from build123d import *

# Parameters (mm, degrees)
SKETCH1_W           = 11.699975178
SKETCH1_H           = 11.699996949
SKETCH1_W_2         = 11.699990436
SKETCH1_H_2         = 11.699981689
SKETCH1_W_3         = 11.699990437
SKETCH1_H_3         = 11.699975177
SKETCH1_W_4         = 11.699981689
SKETCH1_H_4         = 11.699990436
BOSS_EXTRUDE1_DEPTH = 1955.8


with BuildPart() as part:
    # Sketch1 → Boss-Extrude1 (new body)
    with BuildSketch(Plane.XY):
        Polygon((22.500515052, 22.499297556), (-22.499484399, 22.499298105), (-22.499484948, -22.500701346), (-4.249491942, -22.500701568), (-4.249491942, -22.200733242), (-4.24949208, -18.000719999), (-6.799479919, -18.000719999), (-6.799480207, -9.200732353), (-4.799480391, -7.200732362), (4.800525817, -7.200732047), (6.8005258, -9.200731855), (6.800526088, -18.000720263), (4.250507877, -18.000720263), (4.250508015, -22.200733153), (4.250508015, -22.500701672), (22.500514502, -22.500701895), (22.500514725, -4.250714302), (22.200520351, -4.250714302), (18.000507108, -4.25071444), (18.000507108, -6.800702279), (9.200519462, -6.800702567), (7.200519471, -4.800702751), (7.200519156, 4.799303458), (9.200518964, 6.79930344), (18.000507424, 6.799303729), (18.000507424, 4.249285514), (22.200520261, 4.249285652), (22.500514829, 4.249285652), align=None)
        with BuildLine():
            Line((-4.249491247, 17.999291576), (-4.249490956, 22.199304807))
            Line((-4.249490956, 22.199304807), (-3.949472548, 22.199304807))
            Line((-3.949472548, 22.199304807), (-3.481695222, 21.73152644))
            ThreePointArc((-3.481695222, 21.73152644), (-2.670636178, 21.189593132), (-1.713926324, 20.999291428))
            Line((-1.713926324, 20.999291428), (1.714975167, 20.999291428))
            ThreePointArc((1.714975167, 20.999291428), (2.671722509, 21.189608628), (3.482801459, 21.731583767))
            Line((3.482801459, 21.731583767), (3.950490798, 22.199304487))
            Line((3.950490798, 22.199304487), (4.250509108, 22.199304487))
            Line((4.250509108, 22.199304487), (4.250508817, 17.999291575))
            Line((4.250508817, 17.999291575), (6.800527063, 17.999291575))
            Line((6.800527063, 17.999291575), (6.800526453, 9.199302988))
            Line((6.800526453, 9.199302988), (4.800526064, 7.199302969))
            Line((4.800526064, 7.199302969), (-4.799479817, 7.199303635))
            Line((-4.799479817, 7.199303635), (-6.799479854, 9.199304042))
            Line((-6.799479854, 9.199304042), (-6.799479244, 17.999291576))
            Line((-6.799479244, 17.999291576), (-4.249491247, 17.999291576))
        make_face(mode=Mode.SUBTRACT)
        with BuildLine():
            Line((-22.199510888, 4.249285566), (-17.999497356, 4.249285704))
            Line((-17.999497356, 4.249285704), (-17.999497356, 6.79927354))
            Line((-17.999497356, 6.79927354), (-9.199509947, 6.799273828))
            Line((-9.199509947, 6.799273828), (-7.199509956, 4.799274012))
            Line((-7.199509956, 4.799274012), (-7.199509641, -4.800732197))
            Line((-7.199509641, -4.800732197), (-9.199509449, -6.800732179))
            Line((-9.199509449, -6.800732179), (-17.99949762, -6.800732468))
            Line((-17.99949762, -6.800732468), (-17.99949762, -4.250714253))
            Line((-17.99949762, -4.250714253), (-22.199510799, -4.250714391))
            Line((-22.199510799, -4.250714391), (-22.199510799, -3.950696126))
            Line((-22.199510799, -3.950696126), (-21.731790056, -3.48300681))
            ThreePointArc((-21.731790056, -3.48300681), (-21.189814855, -2.671927844), (-20.999497617, -1.71518046))
            Line((-20.999497617, -1.71518046), (-20.999497617, 1.713721031))
            ThreePointArc((-20.999497617, 1.713721031), (-21.189799286, 2.670430863), (-21.731732544, 3.481489907))
            Line((-21.731732544, 3.481489907), (-22.199510888, 3.949267256))
            Line((-22.199510888, 3.949267256), (-22.199510888, 4.249285566))
        make_face(mode=Mode.SUBTRACT)
        with Locations((-14.649542346, -14.650709384)):
            Rectangle(SKETCH1_W, SKETCH1_H, mode=Mode.SUBTRACT)
        with Locations((14.65050626, -14.650767962)):
            Rectangle(SKETCH1_W_2, SKETCH1_H_2, mode=Mode.SUBTRACT)
        with BuildLine():
            Line((-3.181457266, -4.596908447), (-4.595670829, -3.182694885))
            Line((-4.595670829, -3.182694885), (-3.26221457, -1.849238626))
            ThreePointArc((-3.26221457, -1.849238626), (-3.749476751, -0.00071437), (-3.26221457, 1.847809887))
            Line((-3.26221457, 1.847809887), (-4.595670829, 3.181266146))
            Line((-4.595670829, 3.181266146), (-3.181457266, 4.595479708))
            Line((-3.181457266, 4.595479708), (-1.848001007, 3.262023449))
            ThreePointArc((-1.848001007, 3.262023449), (0.000523249, 3.74928563), (1.849047505, 3.262023449))
            Line((1.849047505, 3.262023449), (3.182503764, 4.595479708))
            Line((3.182503764, 4.595479708), (4.596717327, 3.181266146))
            Line((4.596717327, 3.181266146), (3.263261068, 1.847809887))
            ThreePointArc((3.263261068, 1.847809887), (3.750523249, -0.00071437), (3.263261068, -1.849238626))
            Line((3.263261068, -1.849238626), (4.596717327, -3.182694885))
            Line((4.596717327, -3.182694885), (3.182503764, -4.596908447))
            Line((3.182503764, -4.596908447), (1.849047505, -3.263452188))
            ThreePointArc((1.849047505, -3.263452188), (0.000523249, -3.75071437), (-1.848001007, -3.263452188))
            Line((-1.848001007, -3.263452188), (-3.181457266, -4.596908447))
        make_face(mode=Mode.SUBTRACT)
        with Locations((-14.64949028, 14.649335967)):
            Rectangle(SKETCH1_W_3, SKETCH1_H_3, mode=Mode.SUBTRACT)
        with Locations((14.650561583, 14.6492839)):
            Rectangle(SKETCH1_W_4, SKETCH1_H_4, mode=Mode.SUBTRACT)
    extrude(amount=BOSS_EXTRUDE1_DEPTH)


solid = part.part
Check sheet for the modelled part. Datum: model origin and axes. Units: mm. Give positions to 0.01 mm unless a question says otherwise; leave off trailing zeros. Use a Markdown table: item, result. Add a question column.
Q1. Sectioned sample at A-A, the plane z = 1232.5. Give the number of separate pieces and of enclosed holes in the cut face, then the cut area to 3 significant figures.
Q2. Go/stop test with flat-tipped pins: pin 1 (4 mm diameter, centred on x = 5, y = 17.5, fed in from -Z); pin 2 (4 mm diameter, centred on y = 0.5, z = 1364, fed in from +X). Record where each tip stops, or that it passes through.
Q3. Scan lines: line 1 along Y through (x, z) = (-2.5, 138.5); line 2 along X through (y, z) = (19, 223); line 3 along X through (y, z) = (10.5, 1129.5). Record each from-to range of solid material in increasing order. Write a range as [from, to].
Verdict:
| question | item | result |
|---|---|---|
| 1 | separate pieces | 1 |
| 1 | enclosed holes | 7 |
| 1 | area | 715 mm^2 |
| 2 | pin 1 | z = 0 |
| 2 | pin 2 | x = 7.2 |
| 3 | line 1 | [-7.2, -3.92], [3.91, 7.2], [21.13, 22.5] |
| 3 | line 2 | [-22.5, -20.5], [-8.8, -4.25], [4.25, 8.8], [20.5, 22.5] |
| 3 | line 3 | [-22.5, -20.5], [-8.8, -6.8], [6.8, 8.8], [20.5, 22.5] |
